The listing builds one solid part. Answer for the finished solid, in the listing's coordinates (mm). Coordinates: 2 decimals unless noted, no trailing zeros. Order: outer loops, then holes, each group sorted by start corner. A loop starts at its lowest first (then second) coordinate and runs counter-clockwise, first axis right, second up.
```python
from build123d import *

# Parameters (mm, degrees)
SKETCH1_R           = 14.2875
BOSS_EXTRUDE1_DEPTH = 200
CHAMFER1_SIZE       = 1.524
CHAMFER1_SIZE2      = 2.639645431


with BuildPart() as part:
    # Sketch1 → Boss-Extrude1 (new body)
    with BuildSketch(Plane(origin=(0, 0, 0), x_dir=(0, 0, -1), z_dir=(1, 0, 0))):
        Circle(SKETCH1_R)
    extrude(amount=BOSS_EXTRUDE1_DEPTH)

    # Chamfer1
    chamfer1_edges = [part.edges().sort_by_distance(p)[0] for p in [
        (200, 0, 14.2875),
    ]]
    chamfer1_side = [part.faces().sort_by_distance(p)[0] for p in [
        (100, 0, 14.2875),
    ]]
    chamfer(chamfer1_edges, length=CHAMFER1_SIZE, length2=CHAMFER1_SIZE2, reference=chamfer1_side[0])

    # Sketch4 → Revolve1 (revolve)
    with BuildSketch(Plane.XY):
        with BuildLine():
            Line((-20, 0), (20, 0))
            ThreePointArc((20, 0), (0, 20), (-20, 0))
        make_face()
    revolve(axis=Axis((0, 0, 0), (1, 0, 0)))


solid = part.part
```
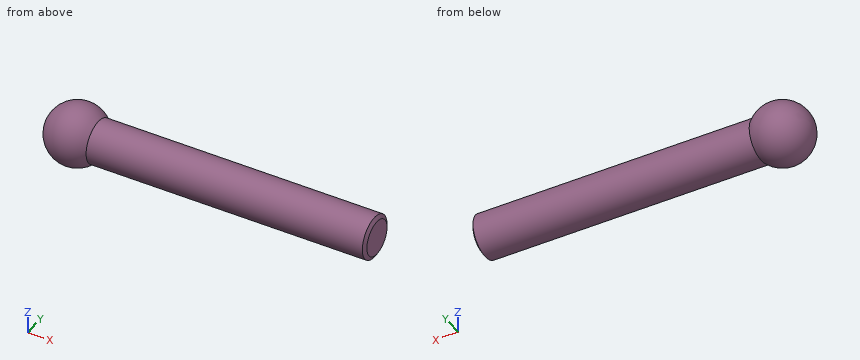
(1) Find section A-A (y = 0). Write down the section's boundary in (x, z).
(2) Consider line 1 (Z direction, x = 114.5, y = 4); line 2 (Y direction, x = 83.5, z = -10.5); line 3 (Y direction, x = 157.5, z = -7). Determine where each line is inside the solid, lowest interval first.
(3) Find section D-D (x = -1). Write down the section's boundary in (y, z), and give its area (3 significant figures).
(4) Find section B-B (x = 68.5). Write down the section's boundary in (y, z) (1 decimal), and give its area (3 significant figures).
(5) Each of these flat-tipped pins is pushed along its axis until it touches: pin 1 Ø3 at (x, y) = (19, 12) entering from -Z; pin 2 Ø8 at (y, z) = (9.5, 2) entering from -X; pin 3 Ø1 at (x, z) = (150.5, 0) entering from +Y; pin 4 Ø12 at (y, z) = (11.5, 4.5) entering from +X. Where does it stop, or does it pass through?
Findings below:
1. outline: (14, -14.29) - (198.48, -14.29) - (200, -11.65) - (200, 11.65) - (198.48, 14.29) - (14, 14.29) arc R20 ccw (long way) to start
2. line 1: z = -13.72 to 13.72
2. line 2: y = -9.69 to 9.69
2. line 3: y = -12.46 to 12.46
3. outline: circle Ø39.95 at (0, 0)
3. area: 1,250 mm2
4. outline: circle Ø28.6 at (0, 0)
4. area: 641 mm2
5. pin 1: stops at z = -9.69
5. pin 2: stops at x = -19.17
5. pin 3: stops at y = 14.29
5. pin 4: stops at x = 200
